```python
from build123d import *

# Parameters (mm, degrees)
SKETCH_1_W          = 18
SKETCH_1_H          = 33.5
EXTRUDE_1_DEPTH     = 1.5
FILLET_1_R          = 1.5
SKETCH_2_W          = 1.5
SKETCH_2_H          = 12
EXTRUDE_2_DEPTH     = 6
SKETCH_3_W          = 14.8
SKETCH_3_H          = 1.6
EXTRUDE_3_DEPTH     = 2
FILLET_2_R          = 2
SKETCH_4_R          = 0.856485036
CUT_EXTRUDE_1_DEPTH = 18
SKETCH_5_W          = 12
SKETCH_5_H          = 8
EXTRUDE_4_DEPTH     = 1
FILLET_3_R          = 1
CUT_EXTRUDE_2_DEPTH = 10


with BuildPart() as part:
    # 草图1 → 凸台-拉伸1 (new body)
    with BuildSketch(Plane(origin=(0, 0, 0), x_dir=(1, 0, 0), z_dir=(0, 1, 0))):
        Rectangle(SKETCH_1_W, SKETCH_1_H)
    extrude(amount=EXTRUDE_1_DEPTH)

    # 圆角1
    fillet_1_edges = [part.edges().sort_by_distance(p)[0] for p in [
        (-9, 0.75, -16.75),
        (9, 0.75, -16.75),
        (9, 0.75, 16.75),
        (-9, 0.75, 16.75),
    ]]
    fillet(fillet_1_edges, radius=FILLET_1_R)

    # 草图2 → 凸台-拉伸2 (add)
    with BuildSketch(Plane(origin=(0, 1.5, 0), x_dir=(1, 0, 0), z_dir=(0, 1, 0))):
        with Locations((-6.65, 7.622409508)):
            Rectangle(SKETCH_2_W, SKETCH_2_H)
        with Locations((6.65, 7.622409508)):
            Rectangle(SKETCH_2_W, SKETCH_2_H)
    extrude(amount=EXTRUDE_2_DEPTH)

    # 草图3 → 凸台-拉伸3 (add)
    with BuildSketch(Plane(origin=(0, 1.5, 0), x_dir=(1, 0, 0), z_dir=(0, 1, 0))):
        with Locations((0, 14.45)):
            Rectangle(SKETCH_3_W, SKETCH_3_H)
    extrude(amount=EXTRUDE_3_DEPTH)

    # 圆角2
    fillet_2_edges = [part.edges().sort_by_distance(p)[0] for p in [
        (-5.9, 1.5, -7.622409508),
        (-6.65, 7.5, -13.622409508),
        (5.9, 1.5, -7.622409508),
        (6.65, 7.5, -13.622409508),
    ]]
    fillet(fillet_2_edges, radius=FILLET_2_R)

    # 草图4 → 切除-拉伸1 (cut)
    with BuildSketch(Plane(origin=(7.4, 0, 0), x_dir=(0, 0, -1), z_dir=(1, 0, 0))):
        with Locations((3.25, 5.5)):
            Circle(SKETCH_4_R)
    extrude(amount=-CUT_EXTRUDE_1_DEPTH, mode=Mode.SUBTRACT)

    # 草图5 → 凸台-拉伸4 (add)
    with BuildSketch(Plane(origin=(0, 1.5, 0), x_dir=(1, 0, 0), z_dir=(0, 1, 0))):
        with Locations((0, -12.75)):
            Rectangle(SKETCH_5_W, SKETCH_5_H)
    extrude(amount=EXTRUDE_4_DEPTH)

    # 圆角3
    fillet_3_edges = [part.edges().sort_by_distance(p)[0] for p in [
        (9, 0, 0),
        (-9, 0, 0),
        (0, 0, -16.75),
        (0, 0, 16.75),
        (-8.560660172, 0, -16.310660172),
        (8.560660172, 0, -16.310660172),
        (-8.560660172, 0, 16.310660172),
        (8.560660172, 0, 16.310660172),
    ]]
    fillet(fillet_3_edges, radius=FILLET_3_R)

    # 草图6 → 切除-拉伸2 (cut)
    with BuildSketch(Plane(origin=(0, 1.5, 0), x_dir=(1, 0, 0), z_dir=(0, 1, 0))):
        Polygon((-6, -16.75), (-6.75, -16.75), (-6.75, -7.75), (-3, -7.75), (-3, -8.75), (-6, -8.75), align=None)
        Polygon((6, -8.75), (6, -16.75), (6.75, -16.75), (6.75, -7.75), (3, -7.75), (3, -8.75), align=None)
    extrude(amount=-CUT_EXTRUDE_2_DEPTH, mode=Mode.SUBTRACT)


solid = part.part
```
The listing builds one solid part. Answer for the finished solid, in the listing's coordinates (mm). A direction names the side the tool comes from. Give positions to 0.01 mm unless a question says otherwise; leave off trailing zeros. Write each loop counter-clockwise with the first axis right and the second up, starting at its lowest first coordinate (ties: lowest second). Pieces come first, ordered by that corner, then holes. Notation, with made-up numbers: M 59,27 L 78,27 A26 cw 78,41 Z; hole C 9.25,47 d8. An arc over 180 degrees is marked long. Write each question's results on one line, items separated by ' | '.
Q1. Section A-A, the plane z = 13.5 is taken. Write down the section's boundary in (x, y), then the cut area to 3 significant figures.
Output values:
outline: M -9,1 A1 ccw -8,0 L -6.75,0 L -6.75,1.5 L -9,1.5 Z; M -6,0 L 6,0 L 6,2.5 L -6,2.5 Z; M 6.75,0 L 8,0 A1 ccw 9,1 L 9,1.5 L 6.75,1.5 Z | area: 36.3 mm2
Q2. Consider L1, parallel to X at y = 1, z = 11.5; L2, parallel to X at y = 3.5, z = -6; L3, parallel to Y at x = -6.5, z = -3.25. Determine where each line is inside the solid, lowest interval first. Write a range as from..to.
Output values:
L1: -9..-6.75, -6..6, 6.75..9 | L2: -7.4..-5.9, 5.9..7.4 | L3: 0..4.64, 6.36..7.5
Q3. A tool of negligible diameter and unlimited length cuts with its end or side. For faces 4 (the flat face through (-3, 1, 8)), 5 (the flat face through (5.9, 5, -8)), 6 (the flat face through (0, 2, -15.25)), 7 (the flat face through (0, 2.5, 13)), from which of +Z, -Z, +X, -X, +Y, -Y can it reach the whole face along a straight path? Write none if from no direction.
Output values:
face 4: +Y, -Y | face 5: +Z, -Z, +Y | face 6: -Z, +X, -X, +Y | face 7: +Z, +X, -X, +Y
Q4. For a pull along Y with two mould halves and no side action, classify faces 1 (the cylindrical face through (-6.64, 4.664, -3.064)), 2 (the cylindrical face through (7.13, 0.301, 16.465)), 3 (the flat face through (7, 7.5, -7)) as released by +Y, released by -Y, zero draft, split by the parting line, or undercut.
Output values:
face 1: undercut | face 2: released by -Y | face 3: released by +Y
Q5. Section B-B, the plane x = -2.25 is taken. Write down the section's boundary in (y, z).
Output values:
outline: M 0,-15.75 A1 ccw 1,-16.75 L 1.5,-16.75 L 1.5,-15.25 L 3.5,-15.25 L 3.5,-13.65 L 1.5,-13.65 L 1.5,8.75 L 2.5,8.75 L 2.5,16.75 L 1,16.75 A1 ccw 0,15.75 Z
Q6. Section C-C, the plane z = 2 is taken. Write down the section's boundary in (x, y), then the cut area to 3 significant figures.
Output values:
outline: M -9,1 A1 ccw -8,0 L 8,0 A1 ccw 9,1 L 9,1.5 L -9,1.5 Z | area: 26.6 mm2
Q7. Flat-ended cylindrical pins translate along their axes: P1, Ø2.5, axis at y = 5.5, z = -3.25, coming from the -X side; P2, Ø3, axis at y = 5.5, z = -9.5, coming from the +X side; P3, Ø4, axis at x = -1, z = 10.5, coming from the +Y side. Find the tip coordinate at first contact, or state that the pin passes through.
Output values:
P1: x = -7.4 | P2: x = 7.4 | P3: y = 2.5
